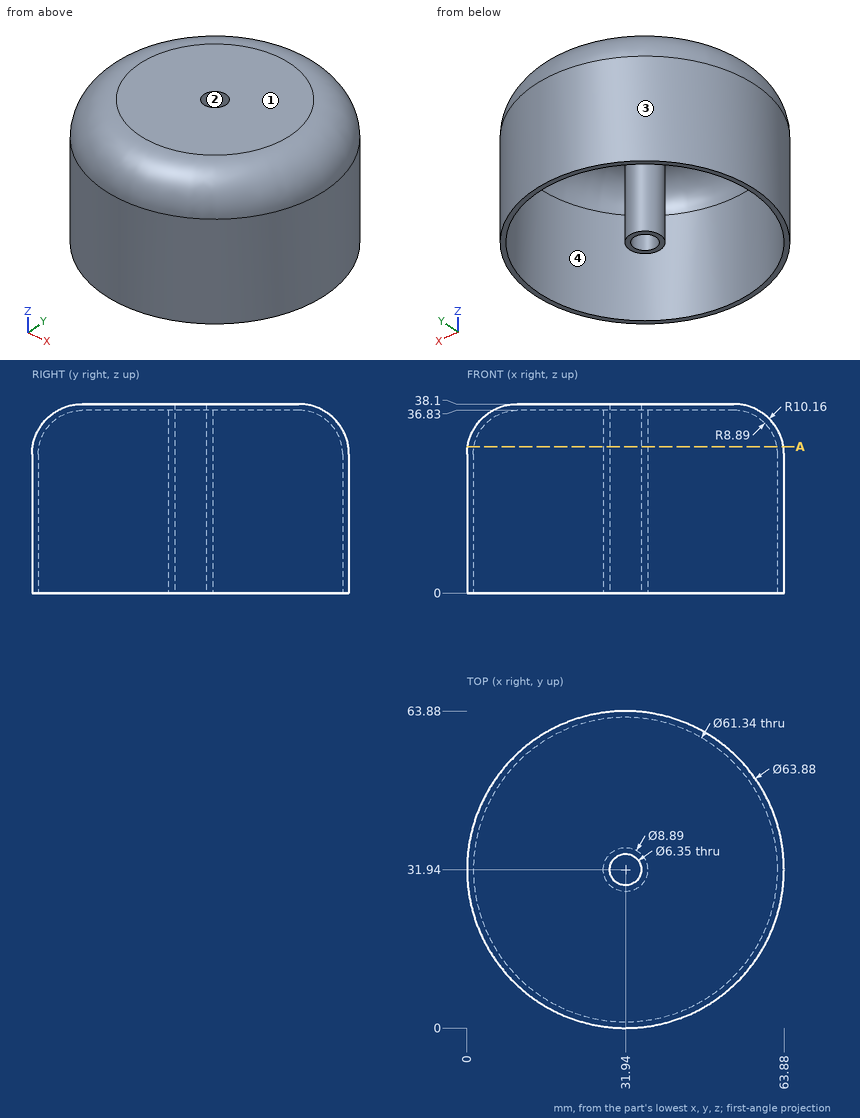
Here's the drawing with two shaded views (mm, measured from the low corner). I have some questions. Round coordinates to 2 decimals unless told otherwise and drop trailing zeros.
1. Suppose I cut it at A-A, the plane z = 29.5. Give the number of separate pieces and of enclosed holes in the cut face.
Answers:
separate pieces: 2
enclosed holes: 2
2. If I drill on probe 1 along Y at (x, z) = (32, 27) (1 decimal); probe 2 along X at (y, z) = (31, 23) (1 decimal); probe 3 along Z at (x, y) = (48, 41.5), over which ranges is the centre line in solid material (lowest first)?
Answers:
probe 1: y = 0 to 1.3, 27.5 to 28.8, 35.1 to 36.4, 62.6 to 63.9
probe 2: x = 0 to 1.3, 27.6 to 28.9, 35 to 36.3, 62.6 to 63.9
probe 3: z = 36.83 to 38.1
3. Will these pins go through, and if not, where does the flat tip stop? pin 1 (5 mm diameter, centred on y = 18, z = 34, fed in from -X); pin 2 (5 mm diameter, centred on y = 25, z = 33, fed in from +X); pin 3 (8 mm diameter, centred on x = 14, z = 24.5, fed in from +Y).
Answers:
pin 1: stops at x = 3.44
pin 2: stops at x = 62.94
pin 3: stops at y = 60.68
4. Thinking about a two-plate mould opening in X: for the marked faces 1, 2, 3 and 4, which applies, released by +X, released by -X, zero draft, split by the parting line, or undercut?
Answers:
face 1: zero draft
face 2: undercut
face 3: split by the parting line
face 4: undercut
